```python
from build123d import *

# Parameters (mm, degrees)
SKETCH1_W                = 171.45
SKETCH1_H                = 171.45
SKETCH1_R                = 1.54305
BOSS_EXTRUDE1_DEPTH      = 8.73125
SKETCH1_3_W              = 171.45
SKETCH1_3_H              = 171.45
SKETCH1_3_R              = 3.175
SKETCH1_3_R_2            = 76.99375
SKETCH1_3_R_3            = 3.3
BOSS_EXTRUDE2_DEPTH      = 9.525
SKETCH1_4_R              = 3.3
BOSS_EXTRUDE3_DEPTH      = 18.3515
CUT_EXTRUDE1_START       = -8.810843
SKETCH2_R                = 3.5
CUT_EXTRUDE1_DEPTH       = 8.810843
CIRPATTERN1_COUNT        = 4
SKETCH1_5_R              = 1.54305
BOSS_EXTRUDE4_DEPTH      = 8.73125
BOSS_EXTRUDE4_DEPTH_BACK = 9.525


with BuildPart() as part:
    # Sketch1 → Boss-Extrude1 (new body)
    with BuildSketch(Plane.XY):
        Rectangle(SKETCH1_W, SKETCH1_H)
        with Locations((0, 25.4)):
            Circle(SKETCH1_R, mode=Mode.SUBTRACT)
    extrude(amount=BOSS_EXTRUDE1_DEPTH)

    # Sketch1<3> → Boss-Extrude2 (add)
    with BuildSketch(Plane.XY):
        Rectangle(SKETCH1_3_W, SKETCH1_3_H)
        with Locations((-73.025, -73.025)):
            Circle(SKETCH1_3_R, mode=Mode.SUBTRACT)
        with Locations((73.025, -73.025)):
            Circle(SKETCH1_3_R, mode=Mode.SUBTRACT)
        with Locations((73.025, 73.025)):
            Circle(SKETCH1_3_R, mode=Mode.SUBTRACT)
        with Locations((-73.025, 73.025)):
            Circle(SKETCH1_3_R, mode=Mode.SUBTRACT)
        Circle(SKETCH1_3_R_2, mode=Mode.SUBTRACT)
        Circle(SKETCH1_3_R_3)
    extrude(amount=-BOSS_EXTRUDE2_DEPTH)

    # Sketch1<4> → Boss-Extrude3 (add)
    with BuildSketch(Plane.XY):
        Circle(SKETCH1_4_R)
    extrude(amount=-BOSS_EXTRUDE3_DEPTH)

    # Sketch2 → Cut-Extrude1 (cut)
    with BuildSketch(Plane(origin=(0, 85.725, 0), x_dir=(1, 0, 0), z_dir=(0, 1, 0)).offset(CUT_EXTRUDE1_START)):
        with Locations((0, 4.7625)):
            Circle(SKETCH2_R)
    cut_extrude1 = extrude(amount=CUT_EXTRUDE1_DEPTH, mode=Mode.SUBTRACT)

    # CirPattern1: Cut-Extrude1 ×4 about axis
    cirpattern1_axis = Axis((0, 0, -9.525), (0, 0, 1))
    for i in range(1, CIRPATTERN1_COUNT):
        add(cut_extrude1.rotate(cirpattern1_axis, i * 360 / CIRPATTERN1_COUNT), mode=Mode.SUBTRACT)

    # Sketch1<5> → Boss-Extrude4 (add, two sides)
    with BuildSketch(Plane.XY) as boss_extrude4_sk:
        with Locations((0, 25.4)):
            Circle(SKETCH1_5_R)
    extrude(amount=BOSS_EXTRUDE4_DEPTH)
    extrude(boss_extrude4_sk.sketch, amount=-BOSS_EXTRUDE4_DEPTH_BACK)


solid = part.part
```
The model under review builds one solid part; all positions refer to its coordinate system, in mm. A direction names the side the tool comes from. Round coordinates to 2 decimals unless told otherwise and drop trailing zeros. Loops run counter-clockwise (first coordinate to the right, second up) from the corner with the lowest first, then second, coordinate; pieces in that order, holes last. Notation, with made-up numbers: (62, 46) - (68, 46) arc R20 ccw to (68, 77) - close; hole circle Ø9 at (10.5, 8). An arc over 180 degrees is marked (long way). Write each question's results on one line, items separated by ' | '. Start each with the question number.
Q1. Take a section at C-C on y = 62. Give the boundary of the cut face in (x, z) (3 decimals).
Q2. Draft analysis for pull direction Z (two halves, no side actions). For faces 1 (the cylindrical face through (0.759, -81.258, -1.346)), 2 (the flat face through (-1, 85.725, 0)), 3 (the flat face through (-73, 73, 0)), state which applies: pulls with the +Z half, pulls with the -Z half, needs draft (parallel to the pull), parting line crosses it, or undercut.
Q3. Take a section at D-D on z = -12.5. Give the boundary of the cut face in (x, y), plus the area to 3 significant figures.
Q4. Take a section at A-A on y = 0. Give the boundary of the cut face in (x, z) (1 decimal), plus the area to 3 significant figures.
Q5. Tool access review of faces 4 (the flat face through (73, 73, 0)), 5 (the flat face through (0, 0, -18.352)), 6 (the cylindrical face through (1.62, 81.26, -1.66)): name each direction out of +Z, -Z, +X, -X, +Y, -Y from which nothing blocks a thin tool from reaching the whole face with its end or side.
Q6. Take a section at B-B on x = -58.5. Give the boundary of the cut face in (y, z) (3 decimals).
Q7. Insertion check: P1, Ø3.5, axis at x = 0.5, y = 25.5, coming from the -Z side (3 decimals); P2, Ø1.9, axis at x = -72.5, y = 73.5, coming from the -Z side; P3, Ø6, axis at y = 46, z = -11.5, coming from the -X side (3 decimals); P4, Ø6.5, axis at x = 0, z = -4.76, coming from the +Y side. Each pin has a flat end and moves straight along its axis. Give the tip position at first contact, or say it passes through.
Q8. Wall thickness on line 1 along Z through (x, y) = (0, -83) (1 decimal); line 2 along X through (y, z) = (71.5, -3.25) (3 decimals); line 3 along Z through (x, y) = (77.5, 44) (3 decimals): over which ranges is each line inside the solid? List them lowest first. Write a range as [from, to].
Data:
1) outline: (-85.725, -9.525) - (-45.651, -9.525) - (-45.651, 0) - (45.651, 0) - (45.651, -9.525) - (85.725, -9.525) - (85.725, 8.731) - (-85.725, 8.731) - close
2) face 1: undercut | face 2: needs draft | face 3: pulls with the -Z half
3) outline: circle Ø6.6 at (0, 0) | area: 34.2 mm²
4) outline: (-85.7, -9.5) - (-77, -9.5) - (-77, -8.3) - (-85.7, -8.3) - close; (-85.7, -1.3) - (-77, -1.3) - (-77, 0) - (-3.3, 0) - (-3.3, -18.4) - (3.3, -18.4) - (3.3, 0) - (77, 0) - (77, -1.3) - (85.7, -1.3) - (85.7, 8.7) - (-85.7, 8.7) - close; (77, -9.5) - (85.7, -9.5) - (85.7, -8.3) - (77, -8.3) - close | area: 1,660 mm²
5) face 4: -Z | face 5: -Z, +X, -X, +Y, -Y | face 6: +Y
6) outline: (-85.725, -9.525) - (-50.058, -9.525) - (-50.058, 0) - (50.058, 0) - (50.058, -9.525) - (85.725, -9.525) - (85.725, 8.731) - (-85.725, 8.731) - close
7) P1: stops at z = -9.525 | P2: stops at z = 0 | P3: stops at x = -85.725 | P4: stops at y = 26.94
8) line 1: z = [-9.5, -8.3], [-1.3, 8.7] | line 2: x = [-85.725, -75.81], [-70.24, -28.562], [28.562, 70.24], [75.81, 85.725] | line 3: z = [-9.525, 8.731]
